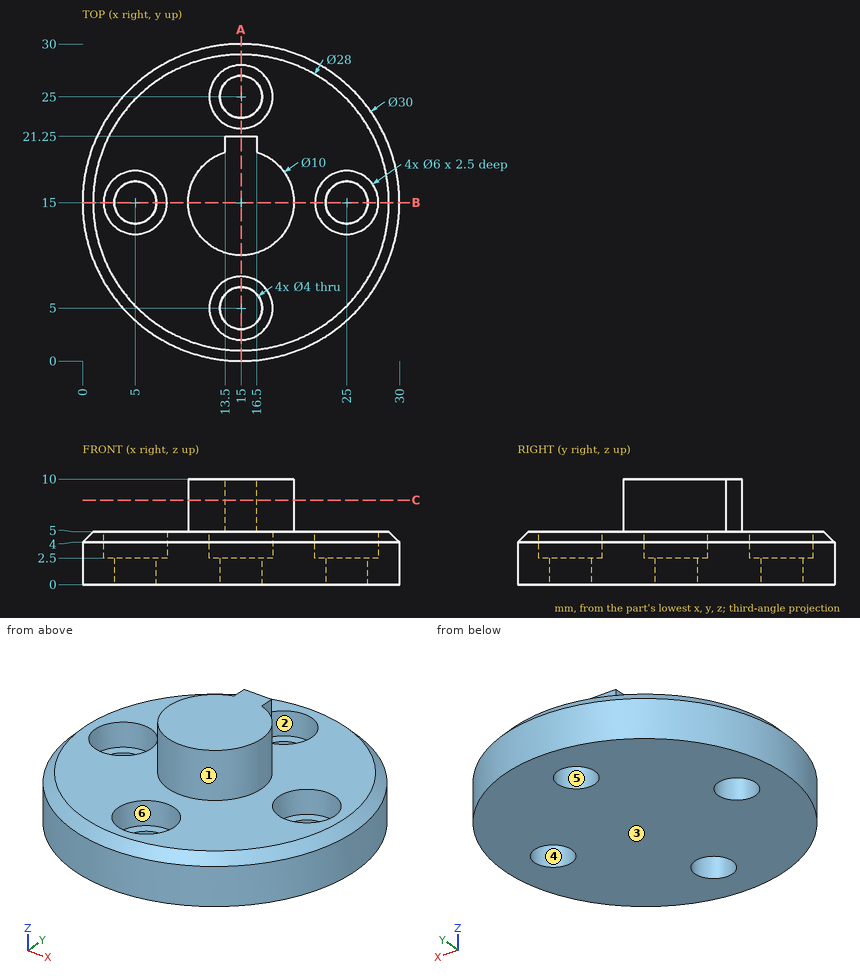
Geometry check sheet. Reference: drawing and pictorial views, mm from the part's lowest x, y, z. A direction names the side the tool comes from. Round coordinates to 2 decimals unless told otherwise and drop trailing zeros. Loops run counter-clockwise (first coordinate to the right, second up) from the corner with the lowest first, then second, coordinate; pieces in that order, holes last. Notation, with made-up numbers: M 26,23.25 L 41,23.25 A21 ccw 41,27.25 Z; hole C 23,-21 d3. An arc over 180 degrees is marked long. Return JSON: item names as keys, results as strings. Group by question number.
(1) Mould release check, pull along X, two halves, no side actions. Record for the marked faces 1, 2, 3 and 4: pulls with the +X half, pulls with the -X half, needs draft (parallel to the pull), parting line crosses it, or undercut.
(2) Set-up check for the marked faces 5 and 6: record each of +Z, -Z, +X, -X, +Y, -Y from which the full face is reachable in a straight line by a thin tool's end or side.
(3) Section check A-A, the plane x = 15. Enter the section's corners in (y, z).
(4) Section check C-C, the plane z = 8. Enter the section's corners in (x, y).
(5) Go/stop test with flat-tipped pins: pin 1 (1.6 mm diameter, centred on y = 21, z = 7, fed in from -X); pin 2 (5 mm diameter, centred on x = 16.5, y = 26, fed in from +Z); pin 3 (0.9 mm diameter, centred on x = 15, z = 8.5, fed in from +Y). Record where each tip stops, or that it passes through.
(6) Scan lines: line 1 along Y through (x, z) = (15, 1.95); line 2 along X through (y, z) = (15.5, 3); line 3 along Z through (x, y) = (23.5, 9.25). Record each from-to range of solid material in increasing order. Write a range as [from, to].
(7) Section check B-B, the plane y = 15. Enter the section's corners in (x, z), and give its area (3 significant figures).
Data:
{
 "1": {"face 1": "parting line crosses it", "face 2": "undercut", "face 3": "needs draft", "face 4": "undercut"},
 "2": {"face 5": "+Z, -Z", "face 6": "+Z"},
 "3": {"outline": "M 0,0 L 3,0 L 3,2.5 L 2,2.5 L 2,5 L 1,5 L 0,4 Z; M 7,0 L 23,0 L 23,2.5 L 22,2.5 L 22,5 L 21.25,5 L 21.25,10 L 10,10 L 10,5 L 8,5 L 8,2.5 L 7,2.5 Z; M 27,0 L 30,0 L 30,4 L 29,5 L 28,5 L 28,2.5 L 27,2.5 Z"},
 "4": {"outline": "M 13.5,19.77 A5 ccw long 16.5,19.77 L 16.5,21.25 L 13.5,21.25 Z"},
 "5": {"pin 1": "x = 13.5", "pin 2": "z = 5", "pin 3": "y = 21.25"},
 "6": {"line 1": "[0, 3], [7, 23], [27, 30]", "line 2": "[0.01, 2.04], [7.96, 22.04], [27.96, 29.99]", "line 3": "[0, 5]"},
 "7": {"outline": "M 0,0 L 3,0 L 3,2.5 L 2,2.5 L 2,5 L 1,5 L 0,4 Z; M 7,0 L 23,0 L 23,2.5 L 22,2.5 L 22,5 L 20,5 L 20,10 L 10,10 L 10,5 L 8,5 L 8,2.5 L 7,2.5 Z; M 27,0 L 30,0 L 30,4 L 29,5 L 28,5 L 28,2.5 L 27,2.5 Z", "area": "149 mm²"}
}
